Can you work these out from the model? Positions are in its coordinate system, mm. Face numbers are marked on the shaded views. A direction names the side the tool comes from. Round coordinates to 2 decimals unless told otherwise and drop trailing zeros. Order: outer loops, then holes, each group sorted by start corner. A loop starts at its lowest first (then second) coordinate and runs counter-clockwise, first axis right, second up. Notation, with made-up numbers: (-7.75, -28.75) - (21.25, -28.75) arc R16 ccw to (21.25, -20.75) - close; hole circle Ø11 at (-2, 37.5). An arc over 180 degrees is marked (long way). Write item = value, one per line.
from build123d import *

# Parameters (mm, degrees)
F0_R     = 31.5
F1_DEPTH = 28
F2_SIZE2 = 20
F2_SIZE  = 7.2794046853
F3_SIZE  = 5
F4_R     = 10
F5_DEPTH = 4
F6_R     = 3
F7_DEPTH = 25


with BuildPart() as f1:
    # F0 (on Front) → F1 (new body)
    with BuildSketch(Plane.XZ):
        Circle(F0_R)
    extrude(amount=F1_DEPTH)

    # F2
    f2_edges = [f1.edges().sort_by_distance(p)[0] for p in [
        (-31.5, -28, 0),
    ]]
    f2_side = f1.faces().sort_by_distance((-31.5, -14, 0))[0]
    chamfer(f2_edges, length=F2_SIZE, length2=F2_SIZE2, reference=f2_side)

    # F3
    f3_edges = [f1.edges().sort_by_distance(p)[0] for p in [
        (-31.5, 0, 0),
    ]]
    chamfer(f3_edges, length=F3_SIZE)

    # F4 (on face) → F5 (join)
    with BuildSketch(Plane.XZ.offset(28)):
        Circle(F4_R)
    extrude(amount=F5_DEPTH)

    # F6 (on face) → F7 (join)
    with BuildSketch(Plane.XZ.offset(32)):
        Circle(F6_R)
    extrude(amount=F7_DEPTH)


solid = f1.part
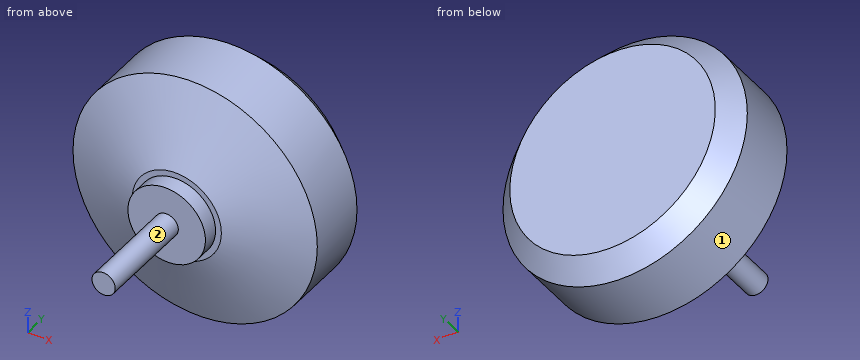
(1) If we section it at C-C (y = -47): Write out the boundary of the cut face in (x, z), plus the area to 3 significant figures.
Computed:
outline = circle Ø6 at (0, 0)
area = 28.3 mm^2
(2) Will these pins go through, and if not, where does the flat tip stop? P1, Ø6, axis at x = -13, z = -1, coming from the -Y side; P2, Ø7, axis at x = -5.5, z = -5.5, coming from the -Y side; P3, Ø3, axis at x = 1.5, y = -42, coming from the +Z side.
Computed:
P1 = -28
P2 = -32
P3 = 3
(3) On a 3-axis mill with a long thin cutter (end or side, diameter ignored), from which of +Z, -Z, +X, -X, +Y, -Y can I reach the whole of each face in a straight line? I mean the marked faces 1 and 2. Say none if no direction works.
Computed:
face_1 = +Y, -Y
face_2 = -Y
(4) If we section it at A-A (z = 0): Write out the boundary of the cut face in (x, y), plus the area to 3 significant figures.
Computed:
outline = (-31.5, -20.72) - (-11.5, -28) - (-10, -28) - (-10, -32) - (-3, -32) - (-3, -57) - (3, -57) - (3, -32) - (10, -32) - (10, -28) - (11.5, -28) - (31.5, -20.72) - (31.5, -5) - (26.5, 0) - (-26.5, 0) - (-31.5, -5) - close
area = 1,820 mm^2
(5) If I drill on line 1 (Z direction, x = -0.5, y = -12.5); line 2 (Y direction, x = -5.5, z = -8); line 3 (Y direction, x = 21.5, z = 2.5), over which ranges is the centre line in solid material (lowest first)? Write a range as from..to.
Computed:
line_1 = -31.5..31.5
line_2 = -32..0
line_3 = -24.31..0
(6) If we section it at D-D (y = -6.5): Write out the boundary of the cut face in (x, z), plus the area to 3 significant figures.
Computed:
outline = circle Ø63 at (0, 0)
area = 3,120 mm^2
(7) If we section it at B-B (x = 0): Write out the boundary of the cut face in (y, z), plus the area to 3 significant figures.
Computed:
outline = (-57, -3) - (-32, -3) - (-32, -10) - (-28, -10) - (-28, -11.5) - (-20.72, -31.5) - (-5, -31.5) - (0, -26.5) - (0, 26.5) - (-5, 31.5) - (-20.72, 31.5) - (-28, 11.5) - (-28, 10) - (-32, 10) - (-32, 3) - (-57, 3) - close
area = 1,820 mm^2
